Autodesk Inventor part; units mm, degrees
ref_plane "YZ Plane" through (0, 0, 0) normal (1, 0, 0) x (0, 1, 0)
ref_plane "XZ Plane" through (0, 0, 0) normal (0, 1, 0) x (-1, 0, 0)
ref_plane "XY Plane" through (0, 0, 0) normal (0, 0, 1) x (1, 0, 0)
sketch "Эскиз1" plane through (0, 0, 0) normal (0, 1, 0) x (-1, 0, 0)
  circle A0 centre (-10.2546, 8.7513) radius 1.3
  circle A1 centre (-4.7546, 9.2513) radius 1.05
  circle A2 centre (-10.2546, 0.7513) radius 1.3
  circle A3 centre (-10.2546, -7.2487) radius 1.3
  circle A4 centre (-4.7546, -6.7487) radius 1.05
  circle A5 centre (11.2454, 9.2513) radius 1.05
  line L0 (-6.7546, 3.1513) -> (13.2454, 3.1513)
  line L1 (-6.7546, -3.3987) -> (-6.7546, 3.1513)
  line L2 (13.2454, -3.3987) -> (-6.7546, -3.3987)
  line L3 (13.2454, 3.1513) -> (13.2454, -3.3987)
  line L4 (3.2454, 3.1513) -> (3.2454, 6.1513)
  line L5 (3.2454, 6.1513) -> (13.2454, 6.1513)
  line L6 (13.2454, 6.1513) -> (13.2454, 11.6513)
  line L7 (13.2454, 11.6513) -> (-12.7546, 11.6513)
  line L8 (-12.7546, 11.6513) -> (-12.7546, -9.3487)
  line L9 (-12.7546, -9.3487) -> (3.2454, -9.3487)
  line L10 (3.2454, -3.3987) -> (3.2454, -6.3987)
  line L11 (3.2454, -6.3987) -> (3.2454, -9.3487)
  line L12 (3.2454, 3.1513) -> (3.2454, -3.3987)
  point P0 (0, 0)
  dimension "d0" = 3
  dimension "d1" = 5.5
  dimension "d2" = 26
  dimension "d3" = 21
  dimension "d4" = 3
extrude "Выдавливание1" add sketch "Эскиз1" along normal blind 3 contours L1 L2 L10 L11 L9 L8 L7 L6 L5 L4 L0 | L0 L12 L2 L1
properties part number "КВ33.044.407 - Заглушка разъема"
Model file for the job. Use its own axes, mm. A direction names the side the tool comes from. Coordinates: 2 decimals unless noted, no trailing zeros. Write each loop counter-clockwise with the first axis right and the second up, starting at its lowest first coordinate (ties: lowest second). Pieces come first, ordered by that corner, then holes. Notation, with made-up numbers: (41.5, -24.5) - (76.5, -24.5) arc R21 cw to (76.5, -3.5) - close; hole circle Ø2 at (-24.75, -19). An arc over 180 degrees is marked (long way). Use a Markdown table: item, result. Add a question column.
Item 1: Two-plate mould, pull along Z, no slides. Class faces 1 (the face through (12.755, 1, 1)), 2 (the face through (9.015, 1.479, 0.361)), 3 (the face through (5, 1, -9.349)): pulls with the +Z half, pulls with the -Z half, needs draft (parallel to the pull), parting line crosses it, or undercut.
Item 2: Band-saw the part on A-A, the plane x = -11.5. Write the cut outline in (y, z).
Item 3: Drop flat-ended pins along their axis: pin 1 (3.5 mm diameter, centred on x = 10.25, z = -7.25, fed in from -Y); pin 2 (1.9 mm diameter, centred on x = 4.75, z = 9.25, fed in from +Y); pin 3 (1.5 mm diameter, centred on y = 1, z = -2.5, fed in from -X); pin 4 (1 mm diameter, centred on x = -10.5, y = 2.5, fed in from -Z). Give the stop position or say it passes through.
Item 4: 3-axis set-ups, long thin cutter, end or side, ignore diameter. For faces 4 (the face through (3, 3, 1)), 5 (the face through (-3.245, 1, -1)): which of +Z, -Z, +X, -X, +Y, -Y reach the whole face in a straight line?
Item 5: Band-saw the part on B-B, the plane y = 0.65. Write the cut outline in (x, z), and give its area (3 significant figures).
Item 6: Drill centre lines: line 1 along Z through (x, y) = (9.5, 0.4); line 2 along Z through (x, y) = (9.75, 2.1); line 3 along Z through (x, y) = (4.5, 1.5). Where is each one in solid material? Low to high.
Item 7: Band-saw the part on C-C, the plane z = 4. Write the cut outline in (x, y).
A:
| question | item | result |
|---|---|---|
| 1 | face 1 | needs draft |
| 1 | face 2 | undercut |
| 1 | face 3 | pulls with the -Z half |
| 2 | outline | (0, 6.15) - (3, 6.15) - (3, 8.23) - (0, 8.23) - close; (0, 10.27) - (3, 10.27) - (3, 11.65) - (0, 11.65) - close |
| 3 | pin 1 | stops at y = 0 |
| 3 | pin 2 | passes through |
| 3 | pin 3 | stops at x = -3.25 |
| 3 | pin 4 | stops at z = 6.15 |
| 4 | face 4 | +Z, -Z, +X, -X, +Y |
| 4 | face 5 | -Z, -X, +Y, -Y |
| 5 | outline | (-13.25, 6.15) - (-3.25, 6.15) - (-3.25, -9.35) - (12.75, -9.35) - (12.75, 11.65) - (-13.25, 11.65) - close; hole circle Ø2.1 at (-11.25, 9.25); hole circle Ø2.1 at (4.75, -6.75); hole circle Ø2.1 at (4.75, 9.25); hole circle Ø2.6 at (10.25, -7.25); hole circle Ø2.6 at (10.25, 0.75); hole circle Ø2.6 at (10.25, 8.75) |
| 5 | area | 365 mm² |
| 6 | line 1 | z = -9.35 to -8.31, -6.19 to -0.31, 1.81 to 7.69, 9.81 to 11.65 |
| 6 | line 2 | z = -9.35 to -8.45, -6.05 to -0.45, 1.95 to 7.55, 9.95 to 11.65 |
| 6 | line 3 | z = -9.35 to -7.77, -5.73 to 8.23, 10.27 to 11.65 |
| 7 | outline | (-3.25, 0) - (12.75, 0) - (12.75, 3) - (-3.25, 3) - close |
